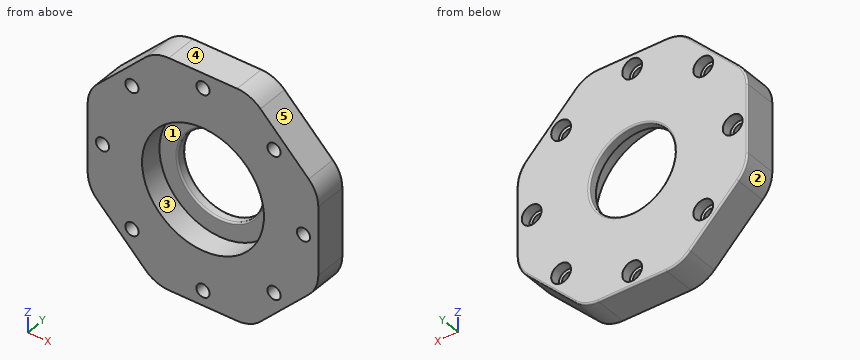
```python
from build123d import *

# Parameters (mm, degrees)
SKETCH1_R           = 32
BOSS_EXTRUDE1_DEPTH = 10
CUT_EXTRUDE1_START  = -10
SKETCH2_R           = 18.5
CUT_EXTRUDE1_DEPTH  = 7
SKETCH3_R           = 13
CUT_EXTRUDE2_DEPTH  = 46.793012567
FILLET2_R           = 0.5
SKETCH6_R           = 32
BOSS_EXTRUDE2_DEPTH = 10
SKETCH7_R           = 2
CUT_EXTRUDE5_DEPTH  = 51.497524692
FILLET3_R           = 0.5
SKETCH8_R           = 3
CUT_EXTRUDE6_DEPTH  = 3
SKETCH5_R           = 2
CUT_EXTRUDE7_DEPTH  = 51.49752483
SKETCH9_R           = 3
CUT_EXTRUDE8_DEPTH  = 3


with BuildPart() as part:
    # Sketch1 → Boss-Extrude1 (new body)
    with BuildSketch(Plane(origin=(0, 0, 0), x_dir=(1, 0, 0), z_dir=(0, 1, 0))):
        with Locations(Location((0, 0, 0), (0, 0, 270))):
            Circle(SKETCH1_R)
    extrude(amount=BOSS_EXTRUDE1_DEPTH)

    # Sketch2 → Cut-Extrude1 (cut)
    with BuildSketch(Plane(origin=(0, 10, 0), x_dir=(1, 0, 0), z_dir=(0, 1, 0)).offset(CUT_EXTRUDE1_START)):
        with Locations(Location((0, 0, 0), (0, 0, 270))):
            Circle(SKETCH2_R)
    extrude(amount=CUT_EXTRUDE1_DEPTH, mode=Mode.SUBTRACT)

    # Sketch3 → Cut-Extrude2 (cut, through all)
    with BuildSketch(Plane(origin=(0, 7, 0), x_dir=(-1, 0, 0), z_dir=(0, -1, 0))):
        with Locations(Location((0, 0, 0), (0, 0, 90))):
            Circle(SKETCH3_R)
    extrude(amount=-CUT_EXTRUDE2_DEPTH, mode=Mode.SUBTRACT)

    # Fillet2
    fillet2_edges = [part.edges().sort_by_distance(p)[0] for p in [
        (0, 10, 13),
        (0, 7, 13),
    ]]
    fillet(fillet2_edges, radius=FILLET2_R)

    # Sketch6 → Boss-Extrude2 (add)
    with BuildSketch(Plane(origin=(0, 0, 0), x_dir=(1, 0, 0), z_dir=(0, 1, 0))):
        with BuildLine():
            Line((10.355339059, 35), (-10.355339059, 35))
            ThreePointArc((-10.355339059, 35), (-14.182173383, 34.238795325), (-17.426406871, 32.071067812))
            Line((-17.426406871, 32.071067812), (-32.071067812, 17.426406871))
            ThreePointArc((-32.071067812, 17.426406871), (-34.238795325, 14.182173383), (-35, 10.355339059))
            Line((-35, 10.355339059), (-35, -10.355339059))
            ThreePointArc((-35, -10.355339059), (-34.238795325, -14.182173383), (-32.071067812, -17.426406871))
            Line((-32.071067812, -17.426406871), (-17.426406871, -32.071067812))
            ThreePointArc((-17.426406871, -32.071067812), (-14.182173383, -34.238795325), (-10.355339059, -35))
            Line((-10.355339059, -35), (10.355339059, -35))
            ThreePointArc((10.355339059, -35), (14.182173383, -34.238795325), (17.426406871, -32.071067812))
            Line((17.426406871, -32.071067812), (32.071067812, -17.426406871))
            ThreePointArc((32.071067812, -17.426406871), (34.238795325, -14.182173383), (35, -10.355339059))
            Line((35, -10.355339059), (35, 10.355339059))
            ThreePointArc((35, 10.355339059), (34.238795325, 14.182173383), (32.071067812, 17.426406871))
            Line((32.071067812, 17.426406871), (17.426406871, 32.071067812))
            ThreePointArc((17.426406871, 32.071067812), (14.182173383, 34.238795325), (10.355339059, 35))
        make_face()
        Circle(SKETCH6_R, mode=Mode.SUBTRACT)
    extrude(amount=BOSS_EXTRUDE2_DEPTH)

    # Sketch7 → Cut-Extrude5 (cut, through all)
    with BuildSketch(Plane(origin=(0, 10, 0), x_dir=(1, 0, 0), z_dir=(0, 1, 0))):
        with Locations(Location((-21.566756826, 21.566756826, 0), (0, 0, 270))):
            Circle(SKETCH7_R)
        with Locations(Location((21.566756826, 21.566756826, 0), (0, 0, 270))):
            Circle(SKETCH7_R)
        with Locations(Location((21.566756826, -21.566756826, 0), (0, 0, 270))):
            Circle(SKETCH7_R)
        with Locations(Location((-21.566756826, -21.566756826, 0), (0, 0, 270))):
            Circle(SKETCH7_R)
    extrude(amount=-CUT_EXTRUDE5_DEPTH, mode=Mode.SUBTRACT)

    # Fillet3
    fillet3_edges = [part.edges().sort_by_distance(p)[0] for p in [
        (-34.238795325, 10, -14.182173383),
        (-35, 10, 0),
        (-34.238795325, 10, 14.182173383),
        (-24.748737342, 10, 24.748737342),
        (-14.182173383, 10, 34.238795325),
        (0, 10, 35),
        (14.182173383, 10, 34.238795325),
        (24.748737342, 10, 24.748737342),
        (34.238795325, 10, 14.182173383),
        (35, 10, 0),
        (34.238795325, 10, -14.182173383),
        (24.748737342, 10, -24.748737342),
        (14.182173383, 10, -34.238795325),
        (0, 10, -35),
        (-14.182173383, 10, -34.238795325),
        (-24.748737342, 10, -24.748737342),
    ]]
    fillet(fillet3_edges, radius=FILLET3_R)

    # Sketch8 → Cut-Extrude6 (cut)
    with BuildSketch(Plane(origin=(0, 10, 0), x_dir=(1, 0, 0), z_dir=(0, 1, 0))):
        with Locations(Location((-21.566756826, 21.566756826, 0), (0, 0, 270))):
            Circle(SKETCH8_R)
        with Locations(Location((21.566756826, 21.566756826, 0), (0, 0, 270))):
            Circle(SKETCH8_R)
        with Locations(Location((21.566756826, -21.566756826, 0), (0, 0, 270))):
            Circle(SKETCH8_R)
        with Locations(Location((-21.566756826, -21.566756826, 0), (0, 0, 270))):
            Circle(SKETCH8_R)
    extrude(amount=-CUT_EXTRUDE6_DEPTH, mode=Mode.SUBTRACT)

    # Sketch5 → Cut-Extrude7 (cut, through all)
    with BuildSketch(Plane(origin=(0, 10, 0), x_dir=(1, 0, 0), z_dir=(0, 1, 0))):
        with Locations(Location((0, 30.5, 0), (0, 0, 270))):
            Circle(SKETCH5_R)
        with Locations(Location((30.5, 0, 0), (0, 0, 270))):
            Circle(SKETCH5_R)
        with Locations(Location((0, -30.5, 0), (0, 0, 270))):
            Circle(SKETCH5_R)
        with Locations(Location((-30.5, 0, 0), (0, 0, 270))):
            Circle(SKETCH5_R)
    extrude(amount=-CUT_EXTRUDE7_DEPTH, mode=Mode.SUBTRACT)

    # Sketch9 → Cut-Extrude8 (cut)
    with BuildSketch(Plane(origin=(0, 10, 0), x_dir=(1, 0, 0), z_dir=(0, 1, 0))):
        with Locations(Location((-30.5, 0, 0), (0, 0, 270))):
            Circle(SKETCH9_R)
        with Locations(Location((0, 30.5, 0), (0, 0, 270))):
            Circle(SKETCH9_R)
        with Locations(Location((30.5, 0, 0), (0, 0, 270))):
            Circle(SKETCH9_R)
        with Locations(Location((0, -30.5, 0), (0, 0, 270))):
            Circle(SKETCH9_R)
    extrude(amount=-CUT_EXTRUDE8_DEPTH, mode=Mode.SUBTRACT)


solid = part.part
```
Geometry: final body of the model. Coordinates: model frame, mm. Face numbers are marked on the shaded views. A direction names the side the tool comes from. Give positions to 0.01 mm unless a question says otherwise; leave off trailing zeros. Return JSON: item names as keys, results as strings.
Item 1: Pin query (flat end, axial travel): P1, Ø3.5, axis at x = 30.5, z = 0, coming from the -Y side; P2, Ø10, axis at x = 19, z = 3, coming from the -Y side; P3, Ø5, axis at x = 30.5, z = 0, coming from the +Y side; P4, Ø2, axis at y = 3, z = -21, coming from the +X side. Return the tip coordinate at first contact, or that it passes through.
Filled in:
{"P1": "through", "P2": "y = 0", "P3": "y = 7", "P4": "x = 29.5"}
Item 2: Section A-A, the plane z = 0. Count the separate pieces of the cut face and the enclosed holes in it, plus the area to 3 significant figures.
Filled in:
{"separate pieces": "4", "enclosed holes": "0", "area": "271 mm^2"}
Item 3: Line query: line 1 (X direction, y = 5.75, z = 0); line 2 (X direction, y = 8.45, z = 0); line 3 (X direction, y = 8.25, z = 20.5). Output: solid intervals per line, ascending.
Filled in:
{"line 1": "-35 to -32.5, -28.5 to -18.5, 18.5 to 28.5, 32.5 to 35", "line 2": "-35 to -33.5, -27.5 to -13, 13 to 27.5, 33.5 to 35", "line 3": "-29 to -24.37, -18.76 to 18.76, 24.37 to 29"}
Item 4: Mould query, pull axis X, two halves, no side actions, for the marked faces 3, 4 and 5. Classes: released by +X, released by -X, zero draft, split by the parting line, or undercut.
Filled in:
{"face 3": "undercut", "face 4": "zero draft", "face 5": "released by +X"}
Item 5: Access query for the marked faces 1 and 2. Directions: +Z, -Z, +X, -X, +Y, -Y. A direction counts if a zero-diameter tool reaches every point of the face in a straight line with its end or side. Return the directions, or none.
Filled in:
{"face 1": "-Y", "face 2": "-Z, -X, +Y, -Y"}
